Here's how the part is built. I have some questions about the finished solid (model axes, mm). A direction names the side the tool comes from. Coordinates: 2 decimals unless noted, no trailing zeros. Write each loop counter-clockwise with the first axis right and the second up, starting at its lowest first coordinate (ties: lowest second). Pieces come first, ordered by that corner, then holes.
(1) Which directions (+Z, -Z, +X, -X, +Y, -Y) give clear straight access to the entire face, cutting with the end or side of a thin tool? Please do faces 1 (the flat face through (15.05, 15, 2)), 2 (the flat face through (-26, 15, 3)).
(2) Imagine slicing it at B-B, the plane y = 10.5. List the corners of the cut face in (x, z) for me.
(3) Imagine slicing it at C-C, the plane y = -13.5. State how many separate pieces and enclosed holes the cut face has, plus the area to 3 significant figures.
(4) For pin 1 Ø6.5 at (x, y) = (68.5, 18) entering from +Z; pin 2 Ø0.8 at (y, z) = (-10.5, 3.5) entering from +X; pin 3 Ø1.4 at (y, z) = (13, 4.5) entering from -X, each with a flat end and sliding along its axis, tell me the tip position at first contact or that it passes through.
(5) Imagine slicing it at A-A, the plane x = 10. List the corners of the cut face in (y, z) for me.
(6) Please list where these lines run through material, in increasing order: probe 1 along Y at (x, z) = (75.5, 3.4); probe 2 along Y at (x, z) = (-11.5, 3.85); probe 3 along Y at (x, z) = (-31.34, 2.25).
```python
from build123d import *

# Parameters (mm, degrees)
P_IDAT_VYSUNUT_M1_DEPTH                           = 2
SKICA2_W                                          = 154
SKICA2_H                                          = 55
P_IDAT_VYSUNUT_M2_DEPTH                           = 2.8
SKICA3_R                                          = 1.6
SKICA3_W                                          = 30.1
SKICA3_H                                          = 22.2
ODEBRAT_VYSUNUT_M1_DEPTH                          = 5.8
SKICA4_W                                          = 145
SKICA4_H                                          = 22.2
ODEBRAT_VYSUNUT_M2_DEPTH                          = 1.8
SKICA5_W                                          = 2
SKICA5_H                                          = 6
P_IDAT_VYSUNUT_M3_DEPTH                           = 2.8
KU_ELOV_ZAHLOUBEN_PRO_M3_ROUBU_SE_Z_P_D           = 3.4
KU_ELOV_ZAHLOUBEN_PRO_M3_ROUBU_SE_Z_P_CSINK_D     = 6.3
KU_ELOV_ZAHLOUBEN_PRO_M3_ROUBU_SE_Z_P_CSINK_ANGLE = 90


with BuildPart() as part:
    # Skica1 → Přidat vysunutím1 (new body)
    with BuildSketch(Plane.XY):
        with BuildLine():
            Line((-90, 33.5), (90, 33.5))
            ThreePointArc((90, 33.5), (91.767766953, 32.767766953), (92.5, 31))
            Line((92.5, 31), (92.5, -31))
            ThreePointArc((92.5, -31), (91.767766953, -32.767766953), (90, -33.5))
            Line((90, -33.5), (-90, -33.5))
            ThreePointArc((-90, -33.5), (-91.767766953, -32.767766953), (-92.5, -31))
            Line((-92.5, -31), (-92.5, 31))
            ThreePointArc((-92.5, 31), (-91.767766953, 32.767766953), (-90, 33.5))
        make_face()
    extrude(amount=P_IDAT_VYSUNUT_M1_DEPTH)

    # Skica2 → Přidat vysunutím2 (add)
    with BuildSketch(Plane.XY.offset(2)):
        Rectangle(SKICA2_W, SKICA2_H)
    extrude(amount=P_IDAT_VYSUNUT_M2_DEPTH)

    # Skica3 → Odebrat vysunutím1 (cut, through all)
    with BuildSketch(Plane.XY.offset(4.8)):
        with Locations((-20, -13.5)):
            Circle(SKICA3_R)
        with Locations((20, -13.5)):
            Circle(SKICA3_R)
        with Locations((33.34, -13.5)):
            Circle(SKICA3_R)
        with Locations((69.34, -13.5)):
            Circle(SKICA3_R)
        with Locations((-31.34, -13.5)):
            Circle(SKICA3_R)
        with Locations((-71.34, -13.5)):
            Circle(SKICA3_R)
        with BuildLine():
            Line((-39.09, -1.1), (-63.59, -1.1))
            ThreePointArc((-63.59, -1.1), (-66.418427125, -2.271572875), (-67.59, -5.1))
            Line((-67.59, -5.1), (-67.59, -21.9))
            ThreePointArc((-67.59, -21.9), (-66.418427125, -24.728427125), (-63.59, -25.9))
            Line((-63.59, -25.9), (-39.09, -25.9))
            ThreePointArc((-39.09, -25.9), (-36.261572875, -24.728427125), (-35.09, -21.9))
            Line((-35.09, -21.9), (-35.09, -5.1))
            ThreePointArc((-35.09, -5.1), (-36.261572875, -2.271572875), (-39.09, -1.1))
        make_face()
        with BuildLine():
            Line((12.25, -1.1), (-12.25, -1.1))
            ThreePointArc((-12.25, -1.1), (-15.078427125, -2.271572875), (-16.25, -5.1))
            Line((-16.25, -5.1), (-16.25, -21.9))
            ThreePointArc((-16.25, -21.9), (-15.078427125, -24.728427125), (-12.25, -25.9))
            Line((-12.25, -25.9), (12.25, -25.9))
            ThreePointArc((12.25, -25.9), (15.078427125, -24.728427125), (16.25, -21.9))
            Line((16.25, -21.9), (16.25, -5.1))
            ThreePointArc((16.25, -5.1), (15.078427125, -2.271572875), (12.25, -1.1))
        make_face()
        with BuildLine():
            Line((61.09, -3.5), (41.59, -3.5))
            ThreePointArc((41.59, -3.5), (38.761572875, -4.671572875), (37.59, -7.5))
            Line((37.59, -7.5), (37.59, -19.5))
            ThreePointArc((37.59, -19.5), (38.761572875, -22.328427125), (41.59, -23.5))
            Line((41.59, -23.5), (61.09, -23.5))
            ThreePointArc((61.09, -23.5), (63.918427125, -22.328427125), (65.09, -19.5))
            Line((65.09, -19.5), (65.09, -7.5))
            ThreePointArc((65.09, -7.5), (63.918427125, -4.671572875), (61.09, -3.5))
        make_face()
        with Locations((-51.34, 14.8)):
            Rectangle(SKICA3_W, SKICA3_H)
        with Locations((0, 14.8)):
            Rectangle(SKICA3_W, SKICA3_H)
        with Locations((51.34, 14.8)):
            Rectangle(SKICA3_W, SKICA3_H)
    extrude(amount=-ODEBRAT_VYSUNUT_M1_DEPTH, mode=Mode.SUBTRACT)

    # Skica4 → Odebrat vysunutím2 (cut)
    with BuildSketch(Plane.XY.offset(4.8)):
        with Locations((0, 14.8)):
            Rectangle(SKICA4_W, SKICA4_H)
    extrude(amount=-ODEBRAT_VYSUNUT_M2_DEPTH, mode=Mode.SUBTRACT)

    # Skica5 → Přidat vysunutím3 (add)
    with BuildSketch(Plane.XY.offset(2)):
        with Locations((-78, 24.5)):
            Rectangle(SKICA5_W, SKICA5_H)
        with Locations((-78, -24.5)):
            Rectangle(SKICA5_W, SKICA5_H)
        with Locations((78, -24.5)):
            Rectangle(SKICA5_W, SKICA5_H)
        with Locations((78, 24.5)):
            Rectangle(SKICA5_W, SKICA5_H)
    extrude(amount=P_IDAT_VYSUNUT_M3_DEPTH)

    # Kuželové zahloubení pro M3 šroubu se zápustnou hlavou plochou1 (through all)
    with Locations(Plane(origin=(0, 0, 0), x_dir=(-1, 0, 0), z_dir=(0, 0, -1))):
        with Locations((-75.5, -24.5), (-75.5, 24.5), (75.5, 24.5), (75.5, -24.5)):
            CounterSinkHole(KU_ELOV_ZAHLOUBEN_PRO_M3_ROUBU_SE_Z_P_D / 2, KU_ELOV_ZAHLOUBEN_PRO_M3_ROUBU_SE_Z_P_CSINK_D / 2, counter_sink_angle=KU_ELOV_ZAHLOUBEN_PRO_M3_ROUBU_SE_Z_P_CSINK_ANGLE)


solid = part.part
```
Recorded:
1. face 1: +Z, -Z
1. face 2: +Z
2. outline: (-92.5, 0) - (-66.39, 0) - (-66.39, 3) - (-72.5, 3) - (-72.5, 4.8) - (-77, 4.8) - (-77, 2) - (-92.5, 2) - close; (-36.29, 0) - (-15.05, 0) - (-15.05, 3) - (-36.29, 3) - close; (15.05, 0) - (36.29, 0) - (36.29, 3) - (15.05, 3) - close; (66.39, 0) - (92.5, 0) - (92.5, 2) - (77, 2) - (77, 4.8) - (72.5, 4.8) - (72.5, 3) - (66.39, 3) - close
3. separate pieces: 10
3. enclosed holes: 0
3. area: 265 mm2
4. pin 1: stops at z = 3
4. pin 2: stops at x = 77
4. pin 3: stops at x = -77
5. outline: (-33.5, 0) - (-25.9, 0) - (-25.9, 4.8) - (-27.5, 4.8) - (-27.5, 2) - (-33.5, 2) - close; (-1.1, 0) - (3.7, 0) - (3.7, 4.8) - (-1.1, 4.8) - close; (25.9, 0) - (33.5, 0) - (33.5, 2) - (27.5, 2) - (27.5, 4.8) - (25.9, 4.8) - close
6. probe 1: y = -27.5 to -26.2, -22.8 to 22.8, 26.2 to 27.5
6. probe 2: y = -27.5 to -25.9, -1.1 to 3.7, 25.9 to 27.5
6. probe 3: y = -27.5 to -15.1, -11.9 to 27.5
